Could you check a few things on this drawing? It's one solid part, dimensions in mm from its lowest x, y, z. A direction names the side the tool comes from. Coordinates: 2 decimals unless noted, no trailing zeros. Loops run counter-clockwise (first coordinate to the right, second up) from the corner with the lowest first, then second, coordinate; pieces in that order, holes last. Notation, with made-up numbers: M -35,65 L -22,65 A23 cw -22,89 Z; hole C -2,40 d2. An arc over 180 degrees is marked long. Answer as a JSON object with one key per item and string values. Group by question number.
Item 1: Suppose I cut it at B-B (x = 50). Write out the boundary of the cut face in (y, z).
Item 2: Suppose I cut it at D-D (x = 28). Write out the boundary of the cut face in (y, z), then the cut area to 3 significant figures.
Item 3: I'm going to push flat-ended pins straight in: pin 1 Ø13 at (x, y) = (88.99, 37.33) entering from +Z; pin 2 Ø5 at (x, z) = (46.5, 11) entering from -Y; pin 3 Ø1.5 at (x, y) = (42.5, 33.5) entering from +Z; pin 4 Ø12 at (x, z) = (31.5, 2.5) entering from +Y. Where does each tip first touch, or does it pass through?
Item 4: Suppose I cut it at C-C (z = 14.25). Count the separate pieces of the cut face and the enclosed holes in it, then the cut area to 3 significant figures.
Item 5: If I drill on line 1 (Y direction, x = 50, z = 11.5); line 2 (Y direction, x = 27.5, z = 3.5); line 3 (Y direction, x = 52, z = 5.75), over which ranges is the centre line in solid material (lowest first)?
Item 6: Suppose I cut it at A-A (y = 50). Write out the boundary of the cut face in (x, z), then the cut area to 3 significant figures.
Item 7: We'd pull the mould along X, two halves only. Please class the marked faces 3, 4, 5 and 6: +X half, -X half, draft (parallel to the pull), parting line (faces both ways), or undercut.
Item 8: Which directions (+Z, -Z, +X, -X, +Y, -Y) give clear straight access to the entire face, cutting with the end or side of a thin tool? Please do the marked faces 1 and 2.
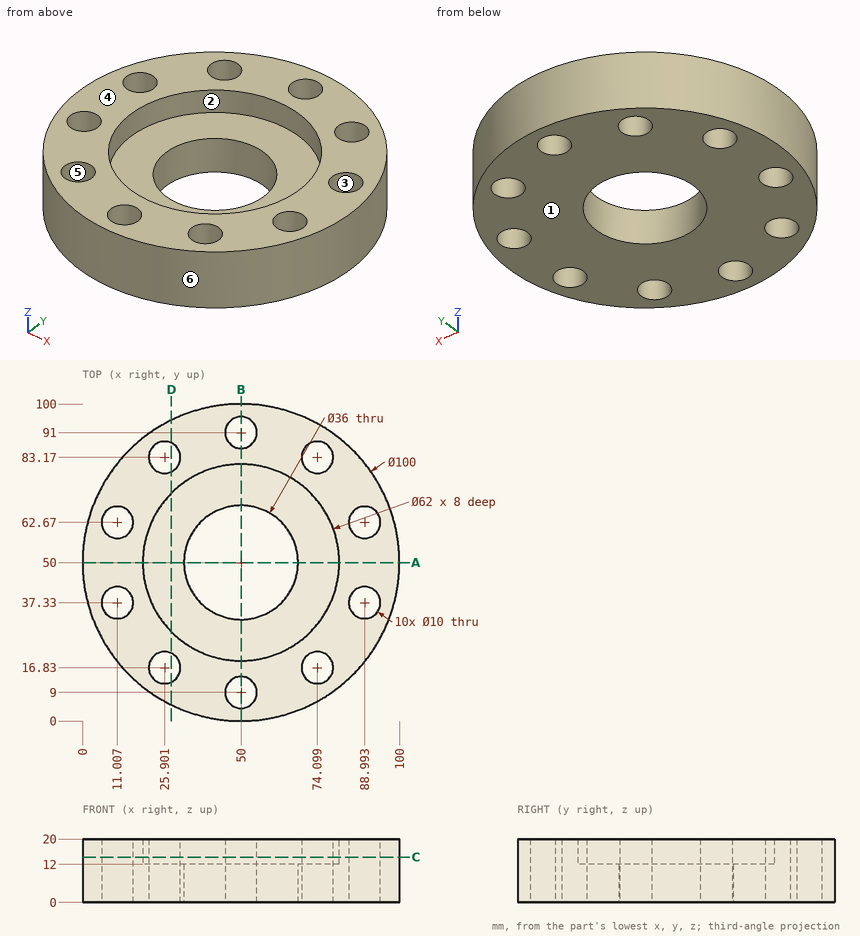
From the geometry:
{
 "1": {"outline": "M 0,0 L 4,0 L 4,20 L 0,20 Z; M 14,0 L 32,0 L 32,12 L 19,12 L 19,20 L 14,20 Z; M 68,0 L 86,0 L 86,20 L 81,20 L 81,12 L 68,12 Z; M 96,0 L 100,0 L 100,20 L 96,20 Z"},
 "2": {"outline": "M 5.1,0 L 12.29,0 L 12.29,20 L 5.1,20 Z; M 21.37,0 L 78.63,0 L 78.63,20 L 71.84,20 L 71.84,12 L 28.16,12 L 28.16,20 L 21.37,20 Z; M 87.71,0 L 94.9,0 L 94.9,20 L 87.71,20 Z", "area": "1,080 mm2"},
 "3": {"pin 1": "z = 20", "pin 2": "y = 0.01", "pin 3": "z = 12", "pin 4": "y = 98.41"},
 "4": {"separate pieces": "1", "enclosed holes": "11", "area": "4,050 mm2"},
 "5": {"line 1": "0 to 4, 14 to 32, 68 to 86, 96 to 100", "line 2": "5.35 to 12.09, 21.57 to 78.43, 87.91 to 94.65", "line 3": "0.04 to 4.42, 13.58 to 32.11, 67.89 to 86.42, 95.58 to 99.96"},
 "6": {"outline": "M 0,0 L 32,0 L 32,12 L 19,12 L 19,20 L 0,20 Z; M 68,0 L 100,0 L 100,20 L 81,20 L 81,12 L 68,12 Z", "area": "1,070 mm2"},
 "7": {"face 3": "undercut", "face 4": "draft", "face 5": "undercut", "face 6": "parting line"},
 "8": {"face 1": "-Z, +X, -X, +Y, -Y", "face 2": "+Z"}
}
